Read the model definition and answer for the solid it produces. Units are mm, in the model's axes. A direction names the side the tool comes from. Coordinates: 2 decimals unless noted, no trailing zeros. Loops run counter-clockwise (first coordinate to the right, second up) from the corner with the lowest first, then second, coordinate; pieces in that order, holes last.
Autodesk Inventor part; units mm, degrees
ref_plane "YZ Plane" through (0, 0, 0) normal (1, 0, 0) x (0, 1, 0)
ref_plane "XZ Plane" through (0, 0, 0) normal (0, 1, 0) x (-1, 0, 0)
ref_plane "XY Plane" through (0, 0, 0) normal (0, 0, 1) x (1, 0, 0)
sketch "Sketch1" plane through (0, 0, 0) normal (0, 1, 0) x (-1, 0, 0)
  circle A0 centre (0, 0) radius 7.75
  circle A1 centre (0, 0) radius 9.25
  dimension "d0" = 15.5
  dimension "d1" = 18.5
extrude "Extrusion1" add sketch "Sketch1" along normal blind 5.5
sketch "Sketch5" plane through (0, 5.5, 0) normal (0, 1, 0) x (1, 0, 0)
  circle A0 centre (0, 0) radius 11.25
  circle A1 centre (0, 0) radius 9
  dimension "d13" = 22.5
  dimension "d14" = 18
extrude "Extrusion5" add sketch "Sketch5" along normal blind 3
move faces "Move1" translate (0, 0.5, 0) faces at (8.4211, 5.5, 1.3362)
properties part number "685ZZFlanged_Adapter_2mm"
Item 1: A cutting plane is placed at A-A on z = 0. Determine the outline of the cut face in (x, y).
Numbers:
outline: (-11.25, 5.5) - (-9.25, 5.5) - (-9.25, 0) - (-7.75, 0) - (-7.75, 6) - (-9, 6) - (-9, 8.5) - (-11.25, 8.5) - close; (7.75, 0) - (9.25, 0) - (9.25, 5.5) - (11.25, 5.5) - (11.25, 8.5) - (9, 8.5) - (9, 6) - (7.75, 6) - close
Item 2: Given pin 1 (9 mm diameter, centred on x = -3.5, z = 0.5, fed in from +Y); pin 2 (1.5 mm diameter, centred on x = -7.5, y = 1.5, fed in from -Z), each flat-ended and moving along its own axis, determine where each tip first touches the part or whether it passes through.
Numbers:
pin 1: stops at y = 6
pin 2: stops at z = -6.32
Item 3: Find the intervals of material crossed by line 1 along Z through (x, y) = (0, 7.4); line 2 along X through (y, z) = (3.3, 0); line 3 along Z through (x, y) = (3.75, 6.5), in increasing order.
Numbers:
line 1: z = -11.25 to -9, 9 to 11.25
line 2: x = -9.25 to -7.75, 7.75 to 9.25
line 3: z = -10.61 to -8.18, 8.18 to 10.61
Item 4: Which of the six approach directions +Z, -Z, +X, -X, +Y, -Y give full straight-line access (tool end or side, diameter ignored) to faces 1 (the face through (-1.172, 7.232, 8.923)), 2 (the face through (-3, 5.5, 9)), 3 (the face through (1.009, 2.958, -7.684))?
Numbers:
face 1: +Y
face 2: -Y
face 3: +Y, -Y
Item 5: A cutting plane is placed at D-D on x = 8.5. Determine the outline of the cut face in (y, z).
Numbers:
outline: (0, -3.65) - (5.5, -3.65) - (5.5, -7.37) - (8.5, -7.37) - (8.5, -2.96) - (6, -2.96) - (6, 2.96) - (8.5, 2.96) - (8.5, 7.37) - (5.5, 7.37) - (5.5, 3.65) - (0, 3.65) - close
Item 6: Determine the mould class of faces 4 (the face through (2.01, 2.71, 9.03)), 5 (the face through (-4, 6, 7)), 6 (the face through (-4, 0, -7)) for opening direction Z: released by +Z, released by -Z, zero draft, split by the parting line, or undercut.
Numbers:
face 4: split by the parting line
face 5: undercut
face 6: zero draft
Item 7: A cutting plane is placed at C-C on y = 3.75. Determine the outline of the cut face in (x, z).
Numbers:
outline: circle Ø18.5 at (0, 0); hole circle Ø15.5 at (0, 0)
Item 8: A cutting plane is placed at B-B on x = 0. Determine the outline of the cut face in (y, z).
Numbers:
outline: (0, -9.25) - (5.5, -9.25) - (5.5, -11.25) - (8.5, -11.25) - (8.5, -9) - (6, -9) - (6, -7.75) - (0, -7.75) - close; (0, 7.75) - (6, 7.75) - (6, 9) - (8.5, 9) - (8.5, 11.25) - (5.5, 11.25) - (5.5, 9.25) - (0, 9.25) - close
